```python
from build123d import *

# Parameters (mm, degrees)
SKETCH1_W           = 50
SKETCH1_H           = 25
SKETCH1_R           = 1.85
BOSS_EXTRUDE1_DEPTH = 1.5
SKETCH2_W           = 50
SKETCH2_H           = 1.5
BOSS_EXTRUDE2_DEPTH = 23.5
SKETCH3_R           = 1.85
CUT_EXTRUDE1_DEPTH  = 23.5
CUT_EXTRUDE2_DEPTH  = 10


with BuildPart() as part:
    # Sketch1 → Boss-Extrude1 (new body)
    with BuildSketch(Plane(origin=(0, 0, 0), x_dir=(1, 0, 0), z_dir=(0, 1, 0))):
        with Locations((25, 12.5)):
            Rectangle(SKETCH1_W, SKETCH1_H)
        with Locations((5, 17.5)):
            Circle(SKETCH1_R, mode=Mode.SUBTRACT)
        with Locations((45, 17.5)):
            Circle(SKETCH1_R, mode=Mode.SUBTRACT)
    extrude(amount=BOSS_EXTRUDE1_DEPTH)

    # Sketch2 → Boss-Extrude2 (add)
    with BuildSketch(Plane.XZ):
        with Locations((25, -0.75)):
            Rectangle(SKETCH2_W, SKETCH2_H)
    extrude(amount=BOSS_EXTRUDE2_DEPTH)

    # Sketch3 → Cut-Extrude1 (cut)
    with BuildSketch(Plane(origin=(0, 0, -1.5), x_dir=(-1, 0, 0), z_dir=(0, 0, -1))):
        with Locations((-20, -19.5)):
            Circle(SKETCH3_R)
        with Locations((-30, -19.5)):
            Circle(SKETCH3_R)
        with Locations((-20, -4.5)):
            Circle(SKETCH3_R)
        with Locations((-30, -4.5)):
            Circle(SKETCH3_R)
    extrude(amount=-CUT_EXTRUDE1_DEPTH, mode=Mode.SUBTRACT)

    # Sketch4 → Cut-Extrude2 (cut)
    with BuildSketch(Plane.XZ):
        with BuildLine():
            Line((50, -8.5), (40, -8.5))
            ThreePointArc((40, -8.5), (37, -5.5), (40, -2.5))
            Line((40, -2.5), (50, -2.5))
            ThreePointArc((50, -2.5), (53, -5.5), (50, -8.5))
        make_face()
    extrude(amount=-CUT_EXTRUDE2_DEPTH, mode=Mode.SUBTRACT)


solid = part.part
```
Model file for the job. Use its own axes, mm. A direction names the side the tool comes from. Give positions to 0.01 mm unless a question says otherwise; leave off trailing zeros. Loops run counter-clockwise (first coordinate to the right, second up) from the corner with the lowest first, then second, coordinate; pieces in that order, holes last. Notation, with made-up numbers: (-22, 55.5) -> (25, 55.5) arc R25 ccw to (25, 74.5) -> close; hole circle Ø11 at (-15, 28.5). An arc over 180 degrees is marked (long way). Use CSV: the item, a comma, the result in double quotes. Start each with the question number.
1) Slice it at D-D on x = 26.5. Give the cut face in (y, z).
2) Tool access for faces 1 (the flat face through (45, 1, -2.5)), 2 (the flat face through (25, -12, -1.5)), 3 (the flat face through (25, 1, -25)): list every direction of +Z, -Z, +X, -X, +Y, -Y with a clear straight run to the whole face (end or side of a thin tool).
3) Mould opens along Y. For faces 4 (the cylindrical face through (21.85, -4.42, -0.76)), 5 (the cylindrical face through (43.636, 0.74, -18.75)), 6 (the flat face through (25, 0, -13)) say: released by +Y, released by -Y, zero draft, split by the parting line, or undercut.
4) Wall check: line 1 (X direction, y = 0.9, z = -17.5); line 2 (Y direction, x = 30, z = -0.45); line 3 (Z direction, x = 45, y = 1.1). Give the ranges that are in metal, low to high.
5) Slice it at B-B on y = -4.5. Give the cut face in (x, z).
6) Flat gauge pins, fed straight in: pin 1 Ø1 at (x, y) = (6.5, -5.5) entering from -Z; pin 2 Ø2 at (y, z) = (-3, -4) entering from +X. Where does each tip first touch, or does it go through?
7) Slice it at C-C on x = 39. Give the cut face in (y, z).
8) Slice it at A-A on x = 45. Give the cut face in (y, z).
Computed values:
1,outline,"(-23.5, -1.5) -> (0, -1.5) -> (0, -25) -> (1.5, -25) -> (1.5, 0) -> (-23.5, 0) -> close"
2,face 1,"+X, +Y, -Y"
2,face 2,"-Z, +X, -X, -Y"
2,face 3,"-Z, +X, -X, +Y, -Y"
3,face 4,"undercut"
3,face 5,"zero draft"
3,face 6,"released by -Y"
4,line 1,"x = 0 to 3.15, 6.85 to 43.15, 46.85 to 50"
4,line 2,"y = -23.5 to -21.35, -17.65 to -6.35, -2.65 to 1.5"
4,line 3,"z = -25 to -19.35, -15.65 to -8.5, -2.5 to 0"
5,outline,"(0, -1.5) -> (18.15, -1.5) -> (18.15, 0) -> (0, 0) -> close; (21.85, -1.5) -> (28.15, -1.5) -> (28.15, 0) -> (21.85, 0) -> close; (31.85, -1.5) -> (50, -1.5) -> (50, 0) -> (31.85, 0) -> close"
6,pin 1,"stops at z = -1.5"
6,pin 2,"passes through"
7,outline,"(-23.5, -1.5) -> (0, -1.5) -> (0, -2.67) -> (1.5, -2.67) -> (1.5, 0) -> (-23.5, 0) -> close; (0, -25) -> (1.5, -25) -> (1.5, -8.33) -> (0, -8.33) -> close"
8,outline,"(-23.5, -1.5) -> (0, -1.5) -> (0, -2.5) -> (1.5, -2.5) -> (1.5, 0) -> (-23.5, 0) -> close; (0, -25) -> (1.5, -25) -> (1.5, -19.35) -> (0, -19.35) -> close; (0, -15.65) -> (1.5, -15.65) -> (1.5, -8.5) -> (0, -8.5) -> close"
